Work out the finished part from the listing and answer in its coordinate system (mm). Face numbers are marked on the shaded views. A direction names the side the tool comes from. Round coordinates to 2 decimals unless told otherwise and drop trailing zeros. Write each loop counter-clockwise with the first axis right and the second up, starting at its lowest first coordinate (ties: lowest second). Pieces come first, ordered by that corner, then holes.
from build123d import *

# Parameters (mm, degrees)
SKETCH1_W                = 25
SKETCH1_H                = 20
BOSS_EXTRUDE1_DEPTH      = 168.81
SKETCH1_W_2              = 20
BOSS_EXTRUDE1_2_DEPTH    = 168.81
CUT_EXTRUDE1_DEPTH       = 194.087721945
CUT_EXTRUDE1_DEPTH_BACK  = 194.087721945
SKETCH2_W                = 25
SKETCH2_H                = 44.708
FILLET2_R                = 10
CUT_EXTRUDE2_DEPTH       = 196.466757701
CUT_EXTRUDE2_DEPTH_BACK  = 196.466757701
SKETCH4_R                = 2.515
CUT_EXTRUDE3_DEPTH       = 186.844513952
CUT_EXTRUDE3_DEPTH_BACK  = 186.844513952
SKETCH3_R                = 2.2
SKETCH5_W                = 58.32
SKETCH5_H                = 66.56
CUT_EXTRUDE4_DEPTH       = 84.405
BOSS_EXTRUDE2_DEPTH      = 7
CHAMFER1_SIZE            = 7
SKETCH8_W                = 20
SKETCH8_H                = 13.858822584
SKETCH8_H_2              = 30.45
CUT_EXTRUDE6_DEPTH       = 2
SKETCH9_W                = 20
SKETCH9_H                = 31.847227872
CUT_EXTRUDE7_DEPTH       = 13
BOSS_EXTRUDE3_START      = -10
SKETCH10_W               = 20
SKETCH10_H               = 10
BOSS_EXTRUDE3_DEPTH      = 30
SKETCH11_W               = 20
SKETCH11_H               = 8.385
BOSS_EXTRUDE4_DEPTH      = 5
CUT_EXTRUDE8_DEPTH       = 135.813629748
CUT_EXTRUDE8_DEPTH_BACK  = 135.813629748
SKETCH12_R               = 1.6
CUT_EXTRUDE11_DEPTH      = 198.714610907
CUT_EXTRUDE11_DEPTH_BACK = 198.714610907
SKETCH13_R               = 1.9
SKETCH14_R               = 3.5
CUT_EXTRUDE12_DEPTH      = 3
CUT_EXTRUDE13_REACH      = 199.715
SKETCH16_W               = 2.468990405
SKETCH16_H               = 10
SKETCH16_W_2             = 2.323465518
SKETCH16_H_2             = 8.385


with BuildPart() as part:
    # Sketch1 → Boss-Extrude1 (new body)
    with BuildSketch(Plane(origin=(0, 0, 0), x_dir=(1, 0, 0), z_dir=(0, 1, 0))):
        Rectangle(SKETCH1_W, SKETCH1_H)
    extrude(amount=BOSS_EXTRUDE1_DEPTH)

    # Sketch2 → Cut-Extrude1 (cut, two sides: drawn at the far end of the back side and taken through both)
    with BuildSketch(Plane.XY.offset(10).offset(-CUT_EXTRUDE1_DEPTH_BACK)):
        with Locations((0, 146.456)):
            Rectangle(SKETCH2_W, SKETCH2_H)
    extrude(amount=CUT_EXTRUDE1_DEPTH + CUT_EXTRUDE1_DEPTH_BACK, mode=Mode.SUBTRACT)

    # Sketch3 → Cut-Extrude3 (cut, two sides: drawn at the far end of the back side and taken through both)
    with BuildSketch(Plane(origin=(12.5, 0, 0), x_dir=(0, 0, -1), z_dir=(1, 0, 0)).offset(-CUT_EXTRUDE3_DEPTH_BACK)):
        with Locations((0, 112.395)):
            Circle(SKETCH3_R)
    extrude(amount=CUT_EXTRUDE3_DEPTH + CUT_EXTRUDE3_DEPTH_BACK, mode=Mode.SUBTRACT)


with BuildPart() as body_2:
    # Sketch1 → Boss-Extrude1 2 (new body)
    with BuildSketch(Plane(origin=(0, 0, 0), x_dir=(1, 0, 0), z_dir=(0, 1, 0))):
        with Locations((63.3814, 38.32)):
            Rectangle(SKETCH1_W_2, SKETCH1_H)
    extrude(amount=BOSS_EXTRUDE1_2_DEPTH)

    # Fillet2
    fillet2_edges = [body_2.edges().sort_by_distance(p)[0] for p in [
        (63.3814, 168.81, -48.32),
        (63.3814, 168.81, -28.32),
    ]]
    fillet(fillet2_edges, radius=FILLET2_R - 0.0001)  # a hair under: the kernel refuses the full size

    # Sketch4 → Cut-Extrude2 (cut, two sides: drawn at the far end of the back side and taken through both)
    with BuildSketch(Plane(origin=(73.3814, 0, 0), x_dir=(0, 0, -1), z_dir=(1, 0, 0)).offset(-CUT_EXTRUDE2_DEPTH_BACK)):
        with Locations((38.32, 156.1084)):
            Circle(SKETCH4_R)
    extrude(amount=CUT_EXTRUDE2_DEPTH + CUT_EXTRUDE2_DEPTH_BACK, mode=Mode.SUBTRACT)


with BuildPart() as cut_extrude4_tool:
    # Sketch5 → Cut-Extrude4 (new, symmetric)
    with BuildSketch(Plane(origin=(12.5, 0, 0), x_dir=(0, 0, -1), z_dir=(1, 0, 0))):
        with Locations((19.16, 33.28)):
            Rectangle(SKETCH5_W, SKETCH5_H)
    extrude(amount=CUT_EXTRUDE4_DEPTH, both=True)


with BuildPart() as part_1:
    add(part.part)

    # Cut-Extrude4: cut by cut_extrude4_tool
    add(cut_extrude4_tool.part, mode=Mode.SUBTRACT)



with BuildPart() as body_2_1:
    add(body_2.part)

    # Cut-Extrude4: cut by cut_extrude4_tool
    add(cut_extrude4_tool.part, mode=Mode.SUBTRACT)


with BuildPart() as part_2:
    add(part_1.part)

    add(body_2_1.part)  # Boss-Extrude2 merges body 2
    # Sketch6 → Boss-Extrude2 (add)
    with BuildSketch(Plane.XZ.offset(-66.56)):
        Polygon((12.5, 10), (-12.5, 10), (-12.5, -48.32), (53.3814, -48.32), (53.3814, -28.32), (73.3814, -28.32), (73.3814, 3.65), (12.5, 3.65), align=None)
    extrude(amount=-BOSS_EXTRUDE2_DEPTH)

    # Chamfer1
    chamfer1_edges = [part_2.edges().sort_by_distance(p)[0] for p in [
        (42.9407, 73.56, 3.65),
    ]]
    chamfer(chamfer1_edges, length=CHAMFER1_SIZE - 0.0001)  # a hair under: the kernel refuses the full size

    # Sketch8 → Cut-Extrude6 (cut)
    with BuildSketch(Plane.ZY.offset(12.5)):
        with Locations((0, 119.324411292)):
            Rectangle(SKETCH8_W, SKETCH8_H)
        with Locations((0, 97.17)):
            Rectangle(SKETCH8_W, SKETCH8_H_2)
    extrude(amount=-CUT_EXTRUDE6_DEPTH, mode=Mode.SUBTRACT)

    # Sketch9 → Cut-Extrude7 (cut)
    with BuildSketch(Plane.ZY.offset(10.5)):
        with Locations((0, 113.318613936)):
            Rectangle(SKETCH9_W, SKETCH9_H)
    extrude(amount=-CUT_EXTRUDE7_DEPTH, mode=Mode.SUBTRACT)

    # Sketch10 → Boss-Extrude3 (add)
    with BuildSketch(Plane.ZY.offset(-2.5).offset(BOSS_EXTRUDE3_START)):
        with Locations((0, 127.645)):
            Rectangle(SKETCH10_W, SKETCH10_H)
    extrude(amount=BOSS_EXTRUDE3_DEPTH)

    # Sketch11 → Boss-Extrude4 (add)
    with BuildSketch(Plane.ZY.offset(12.5)):
        with Locations((0, 77.7525)):
            Rectangle(SKETCH11_W, SKETCH11_H)
    extrude(amount=BOSS_EXTRUDE4_DEPTH)

    # Sketch12 → Cut-Extrude8 (cut, two sides: drawn at the far end of the back side and taken through both)
    with BuildSketch(Plane.XZ.offset(-66.56).offset(-CUT_EXTRUDE8_DEPTH_BACK)):
        with Locations(Location((-0.5, -17, 0), (0, 0, 270))):
            Circle(SKETCH12_R)
        with Locations(Location((46.3814, -41.32, 0), (0, 0, 270))):
            Circle(SKETCH12_R)
        with Locations(Location((66.3814, -10.35, 0), (0, 0, 270))):
            Circle(SKETCH12_R)
        with Locations(Location((-0.5, -41.32, 0), (0, 0, 270))):
            Circle(SKETCH12_R)
    extrude(amount=CUT_EXTRUDE8_DEPTH + CUT_EXTRUDE8_DEPTH_BACK, mode=Mode.SUBTRACT)

    # Sketch13 → Cut-Extrude11 (cut, two sides: drawn at the far end of the back side and taken through both)
    with BuildSketch(Plane.ZY.offset(17.5).offset(-CUT_EXTRUDE11_DEPTH_BACK)):
        with Locations((-5, 127.045)):
            Circle(SKETCH13_R)
        with Locations((5, 127.045)):
            Circle(SKETCH13_R)
        with Locations((5, 77.545)):
            Circle(SKETCH13_R)
        with Locations((-5, 77.545)):
            Circle(SKETCH13_R)
    extrude(amount=CUT_EXTRUDE11_DEPTH + CUT_EXTRUDE11_DEPTH_BACK, mode=Mode.SUBTRACT)

    # Sketch14 → Cut-Extrude12 (cut)
    with BuildSketch(Plane(origin=(12.5, 0, 0), x_dir=(0, 0, -1), z_dir=(1, 0, 0))):
        with Locations((5, 127.045)):
            Circle(SKETCH14_R)
        with Locations((-5, 127.045)):
            Circle(SKETCH14_R)
        with Locations((-5, 77.545)):
            Circle(SKETCH14_R)
        with Locations((5, 77.545)):
            Circle(SKETCH14_R)
    extrude(amount=-CUT_EXTRUDE12_DEPTH, mode=Mode.SUBTRACT)

    # Cut-Extrude13: up to this face of the body (flat: up to its plane)
    cut_extrude13_end = Plane(part_2.part.faces().sort_by_distance((-10.5, 89.67, 0))[0])
    # Sketch16 → Cut-Extrude13 (cut, up to the picked face)
    with BuildSketch(Plane.ZY.offset(17.5), mode=Mode.PRIVATE) as cut_extrude13_sk1:
        with Locations((-0.007149366, 127.645)):
            Rectangle(SKETCH16_W, SKETCH16_H)
    cut_extrude13_tool1 = split(extrude(cut_extrude13_sk1.sketch, amount=-CUT_EXTRUDE13_REACH, mode=Mode.PRIVATE), bisect_by=cut_extrude13_end, keep=Keep.BOTH, mode=Mode.PRIVATE)
    # Sketch16 → Cut-Extrude13 (cut, up to the picked face)
    with BuildSketch(Plane.ZY.offset(17.5), mode=Mode.PRIVATE) as cut_extrude13_sk2:
        with Locations((-0.29586588, 77.7525)):
            Rectangle(SKETCH16_W_2, SKETCH16_H_2)
    cut_extrude13_tool2 = split(extrude(cut_extrude13_sk2.sketch, amount=-CUT_EXTRUDE13_REACH, mode=Mode.PRIVATE), bisect_by=cut_extrude13_end, keep=Keep.BOTH, mode=Mode.PRIVATE)
    add(cut_extrude13_tool1.solids().sort_by(Axis((-17.5, 127.645, -0.007149), (1, 0, 0)))[0], mode=Mode.SUBTRACT)
    add(cut_extrude13_tool2.solids().sort_by(Axis((-17.5, 77.7525, -0.295866), (1, 0, 0)))[0], mode=Mode.SUBTRACT)


solid = part_2.part
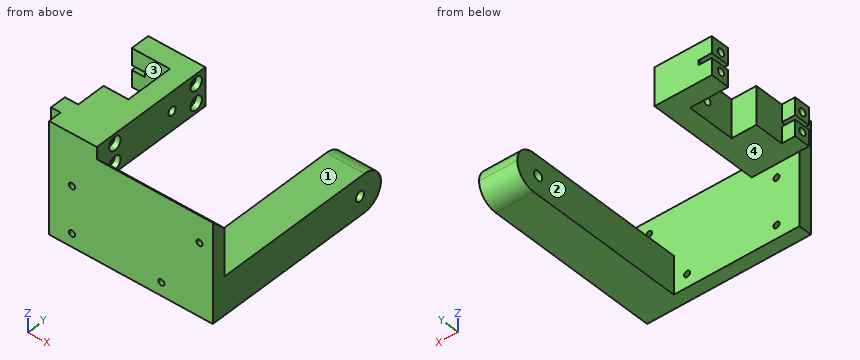
Q1. Find section D-D (z = -17). Determine the outline of the cut face in (x, y).
Q2. Find section C-C (x = -0.5). Determine the outline of the cut face in (y, z) (3 decimals).
Q3. Given pin 1 (6 mm diameter, centred on x = 60, y = 104, fed in from +Z); pin 2 (4 mm diameter, centred on y = 106, z = -6, fed in from +X); pin 3 (6 mm diameter, centred on y = 77.545, z = -5, fed in from +X), each flat-ended and moving along its own axis, determine where each tip first touches the part or whether it passes through.
Q4. Find the intervals of material crossed by L1, parallel to Y at x = 11.15, z = -5 (3 decimals); L2, parallel to Y at x = -2, z = -7 (3 decimals); L3, parallel to Y at x = 41, z = -30, in increasing order.
Q5. Find section B-B (y = 95.5). Determine the outline of the cut face in (x, z), plus the area to 3 significant figures.
Q6. A tool of negligible diameter and unlimited length cuts with its end or side. For the marked faces 1, 2, 3 and 4, from which of +Z, -Z, +X, -X, +Y, -Y can it reach the whole face along a straight path? Write none if from no direction.
Q7. Find section A-A (z = 5). Determine the outline of the cut face in (x, y) (3 decimals).
Report:
1. outline: (-12.5, 66.56) - (-2.1, 66.56) - (-2.1, 73.56) - (-12.5, 73.56) - close; (1.1, 66.56) - (73.38, 66.56) - (73.38, 73.56) - (1.1, 73.56) - close
2. outline: (66.56, -48.32) - (73.56, -48.32) - (73.56, -42.92) - (66.56, -42.92) - close; (66.56, -39.72) - (73.56, -39.72) - (73.56, -18.6) - (66.56, -18.6) - close; (66.56, -15.4) - (73.56, -15.4) - (73.56, -10) - (97.395, -10) - (97.395, 10) - (66.56, 10) - close; (122.645, -10) - (132.645, -10) - (132.645, 10) - (122.645, 10) - close; hole circle Ø3.8 at (77.545, -5); hole circle Ø3.8 at (77.545, 5); hole circle Ø3.8 at (127.045, -5); hole circle Ø3.8 at (127.045, 5)
3. pin 1: stops at z = -28.32
3. pin 2: stops at x = 12.5
3. pin 3: stops at x = 9.5
4. L1: y = 66.56 to 74.045, 81.045 to 123.545, 130.545 to 132.645
4. L2: y = 66.56 to 97.395, 122.645 to 132.645
4. L3: y = 66.56 to 73.56
5. outline: (-10.5, -10) - (12.5, -10) - (12.5, 10) - (-10.5, 10) - close; (53.38, -48.32) - (73.38, -48.32) - (73.38, -28.32) - (53.38, -28.32) - close
5. area: 860 mm2
6. face 1: +Z, +X, -X, +Y
6. face 2: +Z, -Z, -X, +Y
6. face 3: +Z, -Z, -X
6. face 4: -Z, +X, -X, +Y
7. outline: (-17.5, 73.56) - (-12.5, 73.56) - (-12.5, 66.56) - (12.5, 66.56) - (12.5, 74.045) - (9.5, 74.045) - (9.5, 75.645) - (-17.5, 75.645) - close; (-17.5, 79.445) - (9.5, 79.445) - (9.5, 81.045) - (12.5, 81.045) - (12.5, 123.545) - (9.5, 123.545) - (9.5, 125.145) - (-17.5, 125.145) - (-17.5, 122.645) - (2.5, 122.645) - (2.5, 97.395) - (-10.5, 97.395) - (-10.5, 81.945) - (-17.5, 81.945) - close; (-17.5, 128.945) - (9.5, 128.945) - (9.5, 130.545) - (12.5, 130.545) - (12.5, 132.645) - (-17.5, 132.645) - close
